```python
from build123d import *

# Parameters (mm, degrees)
F0_W           = 57.15
F0_H           = 57.15
F1_DEPTH       = 6.35
F3_D           = 4.9784
F3_CSINK_D     = 10.4394
F3_CSINK_ANGLE = 82
F4_R           = 25.4
F4_R_2         = 22.225
F5_DEPTH       = 6.35
F6_R           = 6.35


# Not quite as in the source:
# - a feature names something its author has since deleted; it is built from what else it names


with BuildPart() as f1:
    # F0 (on Top) → F1 (new body)
    with BuildSketch(Plane.XY):
        Rectangle(F0_W, F0_H)
    extrude(amount=F1_DEPTH)

    # F3 (through all)
    with Locations(Plane.XY.offset(6.35)):
        with Locations((-22.225, 22.225), (22.225, 22.225), (22.225, -22.225), (-22.225, -22.225)):
            CounterSinkHole(F3_D / 2, F3_CSINK_D / 2, counter_sink_angle=F3_CSINK_ANGLE)

    # F4 (on face) → F5 (join)
    with BuildSketch(Plane.XY.offset(6.35)):
        Circle(F4_R)
        Circle(F4_R_2, mode=Mode.SUBTRACT)
    extrude(amount=F5_DEPTH)

    # F6
    f6_edges = [f1.edges().sort_by_distance(p)[0] for p in [
        (28.575, 28.575, 3.175),
        (-28.575, 28.575, 3.175),
        (28.575, -28.575, 3.175),
        (-28.575, -28.575, 3.175),
    ]]
    fillet(f6_edges, radius=F6_R)


solid = f1.part
```
Could you check a few things on this model? Use its own coordinates, in mm. A direction names the side the tool comes from. Give positions to 0.01 mm unless a question says otherwise; leave off trailing zeros. Write each loop counter-clockwise with the first axis right and the second up, starting at its lowest first coordinate (ties: lowest second). Pieces come first, ordered by that corner, then holes. Notation, with made-up numbers: (85, -26) -> (107, -26) arc R20 ccw to (107, 6) -> close; hole circle Ø2 at (68.25, 47.5). An arc over 180 degrees is marked (long way). Write each question's results on one line, items separated by ' | '.
1. I need wall thicknesses on L1, parallel to Y at x = 0, z = 10.25 (3 decimals); L2, parallel to Y at x = 23.5, z = 5.75; L3, parallel to X at y = -24.5, z = 5.75. Which ranges of each line are inside material? Lowest first, please.
Check sheet entries:
L1: y = -25.4 to -22.225, 22.225 to 25.4 | L2: y = -28.45 to -26.75, -17.7 to 17.7, 26.75 to 28.45 | L3: x = -28.15 to -26.34, -18.11 to 18.11, 26.34 to 28.15
2. Will these pins go through, and if not, where does the flat tip stop? pin 1 Ø4 at (x, z) = (-8, 11) entering from +Y; pin 2 Ø13.5 at (x, y) = (-6, -5) entering from +Z; pin 3 Ø1 at (x, z) = (13, 9) entering from +Y.
Check sheet entries:
pin 1: stops at y = 24.68 | pin 2: stops at z = 6.35 | pin 3: stops at y = 22.11
3. I want a section at D-D, the plane z = 10.75. Write out the boundary of the cut face in (x, y) (3 decimals), then the cut area to 3 significant figures.
Check sheet entries:
outline: circle Ø50.8 at (0, 0); hole circle Ø44.45 at (0, 0) | area: 475 mm²
4. On a 3-axis mill with a long thin cutter (end or side, diameter ignored), from which of +Z, -Z, +X, -X, +Y, -Y can I reach the whole of each face in a straight line? I mean faces 5 (the flat face through (-15, -21, 6.35)), 6 (the cylindrical face through (26.67, 26.76, 3.22)). Say none if no direction works.
Check sheet entries:
face 5: +Z | face 6: +Z, -Z, +X, +Y
5. I want a section at A-A, the plane z = 1.75. Write out the boundary of the cut face in (x, y) (3 decimals), then the cut area to 3 significant figures.
Check sheet entries:
outline: (-28.575, -22.225) arc R6.35 ccw to (-22.225, -28.575) -> (22.225, -28.575) arc R6.35 ccw to (28.575, -22.225) -> (28.575, 22.225) arc R6.35 ccw to (22.225, 28.575) -> (-22.225, 28.575) arc R6.35 ccw to (-28.575, 22.225) -> close; hole circle Ø4.978 at (-22.225, -22.225); hole circle Ø4.978 at (-22.225, 22.225); hole circle Ø4.978 at (22.225, -22.225); hole circle Ø4.978 at (22.225, 22.225) | area: 3,150 mm²
6. If we mould it in two halves opening along Y, with no side actions, what happens to faces 1 (the cylindrical face through (21.199, 6.676, 9.481)), 2 (the flat face through (-28.575, 0, 3)), 3 (the cylindrical face through (-26.76, 26.67, 3.22)), 4 (the cylindrical face through (20.887, -20.126, 1.582))? For each: released by +Y, released by -Y, zero draft, split by the parting line, or undercut.
Check sheet entries:
face 1: undercut | face 2: zero draft | face 3: released by +Y | face 4: undercut
7. I want a section at B-B, the plane x = 0. Write out the boundary of the cut face in (y, z) (3 decimals), then the cut area to 3 significant figures.
Check sheet entries:
outline: (-28.575, 0) -> (28.575, 0) -> (28.575, 6.35) -> (25.4, 6.35) -> (25.4, 12.7) -> (22.225, 12.7) -> (22.225, 6.35) -> (-22.225, 6.35) -> (-22.225, 12.7) -> (-25.4, 12.7) -> (-25.4, 6.35) -> (-28.575, 6.35) -> close | area: 403 mm²
